Read the model definition and answer for the solid it produces. Units are mm, in the model's axes. Face numbers are marked on the shaded views. A direction names the side the tool comes from. Coordinates: 2 decimals unless noted, no trailing zeros. Loops run counter-clockwise (first coordinate to the right, second up) from the corner with the lowest first, then second, coordinate; pieces in that order, holes last. Notation, with made-up numbers: (61, 2.5) - (107, 2.5) arc R29 cw to (107, 28.5) - close; hole circle Ø10 at (27, -30.5). An arc over 180 degrees is marked (long way). One line per item, written item: value. Start each with the question number.
Autodesk Inventor part; units mm, degrees
ref_plane "YZ Plane" through (0, 0, 0) normal (1, 0, 0) x (0, 1, 0)
ref_plane "XZ Plane" through (0, 0, 0) normal (0, 1, 0) x (-1, 0, 0)
ref_plane "XY Plane" through (0, 0, 0) normal (0, 0, 1) x (1, 0, 0)
sketch "Sketch1" plane through (0, 0, 0) normal (1, 0, 0) x (0, 1, 0)
  line L0 (30, 30) -> (-30, 30)
  line L1 (-30, 30) -> (-30, -30)
  line L2 (-30, -30) -> (30, -30)
  line L3 (30, -30) -> (30, 30)
  line L4 (30, 30) -> (-30, -30) construction
  line L5 (-30, 30) -> (30, -30) construction
  point P0 (0, 0)
  dimension "d0" = 60
  dimension "d1" = 60
extrude "Extrusion1" add sketch "Sketch1" along normal blind 18
fillet "Fillet1" radius 4 4 edges at (9, 30, 30) (9, 30, -30) (9, -30, 30) (9, -30, -30)
sketch "Sketch2" plane through (0, 0, 0) normal (-1, 0, 0) x (0, 0, 1)
  circle A0 centre (0, 0) radius 24.15
  dimension "d5" = 48.3
extrude "Extrusion2" add sketch "Sketch2" along normal blind 0.1
sketch "Sketch3" plane through (-0.1, 0, 0) normal (-1, 0, 0) x (0, 0, 1)
  circle A0 centre (0, 0) radius 23.35
  dimension "d8" = 46.7
extrude "Extrusion3" cut sketch "Sketch3" against normal through all
sketch "Sketch4" plane through (18, 0, 0) normal (1, 0, 0) x (0, 0, -1)
  circle A0 centre (0, 0) radius 24
  dimension "d11" = 48
extrude "Extrusion4" cut sketch "Sketch4" against normal blind 3
sketch "Sketch5" plane through (0, 0, 0) normal (-1, 0, 0) x (0, 0, 1)
  point P0 (0, 0)
sketch "Sketch6" plane through (0, 0, 0) normal (-1, 0, 0) x (0, 0, 1)
  circle A0 centre (23, 17.5) radius 3
  line L0 (30, 26) -> (30, -26)
  line L1 (-26, 30) -> (26, 30)
  circle A1 centre (-23, -17.5) radius 3
  line L2 (-30, -26) -> (-30, 26)
  line L3 (26, -30) -> (-26, -30)
  circle A2 centre (-23.5, 23.5) radius 2.5
  circle A3 centre (23.5, -23.5) radius 2.5
  point P0 (0, 0)
  dimension "d15" = 7
  dimension "d16" = 12.5
  dimension "d17" = 6
  dimension "d18" = 6
  dimension "d19" = 7
  dimension "d20" = 12.5
  dimension "d21" = 23.5
  dimension "d22" = 23.5
  dimension "d23" = 23.5
  dimension "d24" = 23.5
  dimension "d25" = 5
  dimension "d26" = 5
extrude "Extrusion5" cut sketch "Sketch6" against normal through all
sketch "Sketch7" plane through (-0.1, 0, 0) normal (-1, 0, 0) x (0, 0, 1)
  circle A0 centre (-23, -17.5) radius 3
  circle A1 centre (23, 17.5) radius 3
  line L0 (-23, -17.5) -> (23, 17.5) construction
  line L1 (-19.9724, -21.4791) -> (26.0276, 13.5209)
  line L2 (19.9724, 21.4791) -> (-26.0276, -13.5209)
  arc A2 (-26.0276, -13.5209) -> (-19.9724, -21.4791) centre (-23, -17.5) ccw
  arc A3 (26.0276, 13.5209) -> (19.9724, 21.4791) centre (23, 17.5) ccw
  point P0 (0, 0)
  point P1 (0, 0)
  dimension "d29" = 10
extrude "Extrusion6" cut sketch "Sketch7" against normal blind 7
thread "Thread1"
thread "Thread2"
properties part number "Mounting Bracket"
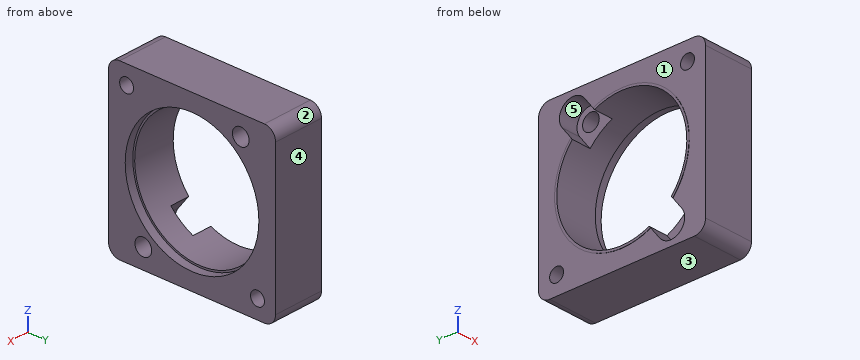
1) Determine the mould class of the marked faces 3, 4 and 5 for opening direction Y: released by +Y, released by -Y, zero draft, split by the parting line, or undercut.
2) Flat-ended cylindrical pins translate along their axes: P1, Ø14, axis at y = -18, z = -23.5, coming from the -X side; P2, Ø4, axis at y = 19.5, z = 24.5, coming from the -X side. Find the tip coordinate at first contact, or state that the pin passes through.
3) Section A-A, the plane x = 14.25 is taken. Determine the outline of the cut face in (y, z).
4) For the marked faces 1 and 2, determine the directions among +Z, -Z, +X, -X, +Y, -Y from which every point of the face is accessible in a straight line to the end or side of a thin tool.
5) Straight lines are drawn through the part: L1, parallel to Y at x = 8, z = 0.5; L2, parallel to Y at x = 10, z = -25.5; L3, parallel to Y at x = 10.25, z = -23.5. For each, find the intervals that lie inside material, in ascending order.
6) Section B-B, the plane z = 0 is taken. Determine the outline of the cut face in (x, y), and give its area (3 significant figures).
7) Section C-C, the plane y = -5 is taken. Determine the outline of the cut face in (x, z).
Answer below:
1. face 3: zero draft
1. face 4: released by +Y
1. face 5: undercut
2. P1: x = 0
2. P2: x = 6.9
3. outline: (-30, -26) arc R4 ccw to (-26, -30) - (26, -30) arc R4 ccw to (30, -26) - (30, 26) arc R4 ccw to (26, 30) - (-26, 30) arc R4 ccw to (-30, 26) - close; hole circle Ø5 at (-23.5, 23.5); hole circle Ø46.7 at (0, 0); hole circle Ø6 at (-17.5, -23); hole circle Ø6 at (17.5, 23); hole circle Ø5 at (23.5, -23.5)
4. face 1: -X
4. face 2: +Z, +X, -X, +Y
5. L1: -30 to -23.34, 23.34 to 30
5. L2: -30 to -19.16, -15.84 to 22, 25 to 30
5. L3: -30 to -20.46, -14.54 to 21, 26 to 30
6. outline: (-0.1, -24.15) - (0, -24.15) - (0, -30) - (18, -30) - (18, -24) - (15, -24) - (15, -23.35) - (-0.1, -23.35) - close; (-0.1, 23.35) - (15, 23.35) - (15, 24) - (18, 24) - (18, 30) - (0, 30) - (0, 24.15) - (-0.1, 24.15) - close
6. area: 236 mm2
7. outline: (-0.1, -23.63) - (0, -23.63) - (0, -30) - (18, -30) - (18, -23.47) - (15, -23.47) - (15, -22.81) - (-0.1, -22.81) - close; (-0.1, 22.81) - (15, 22.81) - (15, 23.47) - (18, 23.47) - (18, 30) - (0, 30) - (0, 23.63) - (-0.1, 23.63) - close
